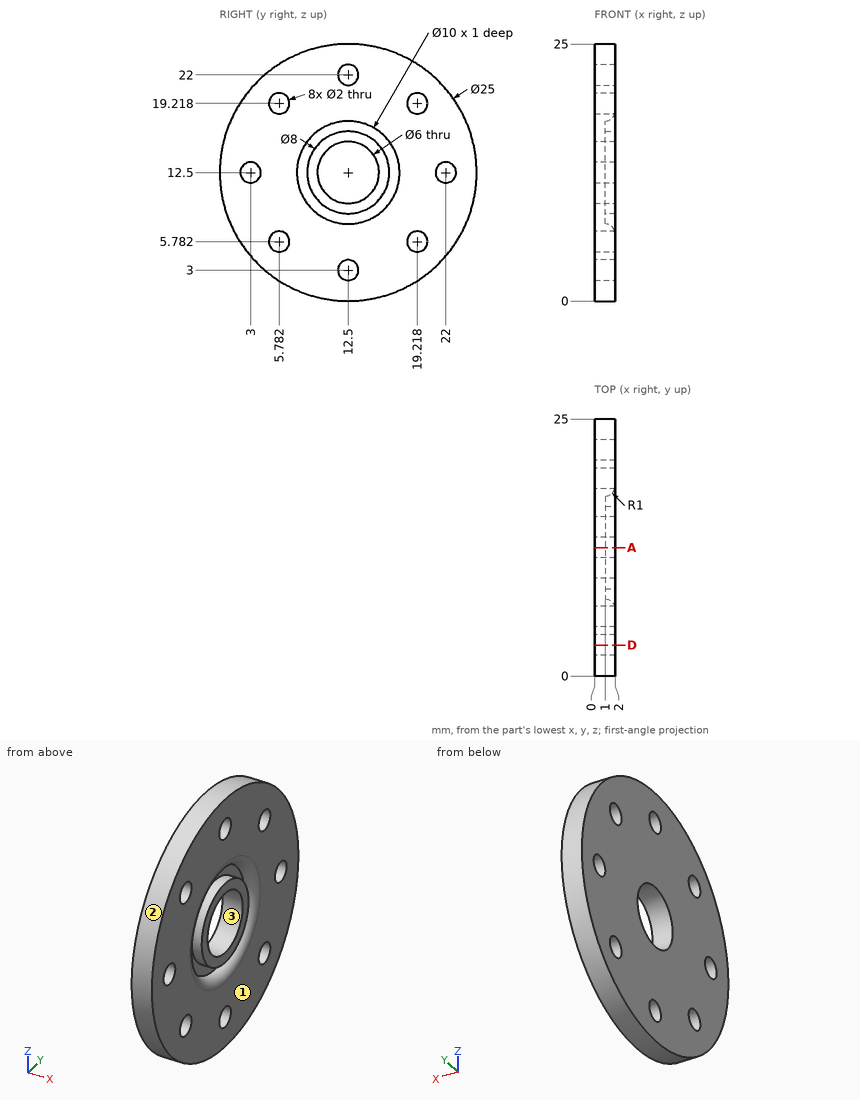
For this review, use the dimensioned drawing (mm, ordinates from the lowest corner) and the shaded views. Give positions to 0.01 mm unless a question says otherwise; leave off trailing zeros. Write each loop counter-clockwise with the first axis right and the second up, starting at its lowest first coordinate (ties: lowest second). Pieces come first, ordered by that corner, then holes. Notation, with made-up numbers: M 32.25,86 L 79.25,86 A8 cw 79.25,93 Z; hole C 65,-9.5 d8. An arc over 180 degrees is marked long. Answer as a JSON object with one key per item and string values. Group by question number.
1) We need section A-A (y = 12.5). Count the separate pieces of the cut face and the enclosed holes in it.
2) Clearance check with flat-ended pins moving along their axes: pin 1 Ø1 at (x, z) = (1.5, 19.5) entering from +Y; pin 2 Ø1 at (x, y) = (0.5, 17) entering from +Z; pin 3 Ø1 at (x, z) = (1, 21.5) entering from +Y (1 decimal). State where each tip first meets the part, or that it passes through.
3) For line 1 along Z through (x, y) = (1.65, 14.5) (1 decimal); line 2 along Z through (x, y) = (1.05, 6.5) (1 decimal); line 3 along Y through (x, z) = (0.6, 12.5), list the stretches that pass through material, from the lowest coordinate up.
4) Mouldability with a two-part tool opening along Y and no side actions: class the marked faces 1, 2 and 3 as released by +Y, released by -Y, zero draft, split by the parting line, or undercut.
5) We need section D-D (y = 3). Give the boundary of the cut face in (x, z) (1 decimal).
Answer key:
{
 "1": {"separate pieces": "4", "enclosed holes": "0"},
 "2": {"pin 1": "stops at y = 23.18", "pin 2": "stops at z = 24.34", "pin 3": "stops at y = 21.7"},
 "3": {"line 1": "z = 0.2 to 7.7, 9 to 10.3, 14.7 to 16, 17.3 to 24.8", "line 2": "z = 1.5 to 5.1, 6.5 to 18.5, 19.9 to 23.5", "line 3": "y = 0 to 2, 4 to 9.5, 15.5 to 21, 23 to 25"},
 "4": {"face 1": "zero draft", "face 2": "split by the parting line", "face 3": "undercut"},
 "5": {"outline": "M 0,4.4 L 2,4.4 L 2,11.5 L 0,11.5 Z; M 0,13.5 L 2,13.5 L 2,20.6 L 0,20.6 Z"}
}
